Geometry: see drawing. Coordinates: mm, zero at the bounding-box minimum. A direction names the side the tool comes from. Give positions to 0.01 mm unless a question says otherwise; leave off trailing zeros. Loops run counter-clockwise (first coordinate to the right, second up) from the corner with the lowest first, then second, coordinate; pieces in that order, holes last. Notation, with made-up numbers: M 63,-12.75 L 100,-12.75 A22 cw 100,16.25 Z; hole C 77,-1 d3. An arc over 180 degrees is marked long. Answer in a Markdown table with one row per item.
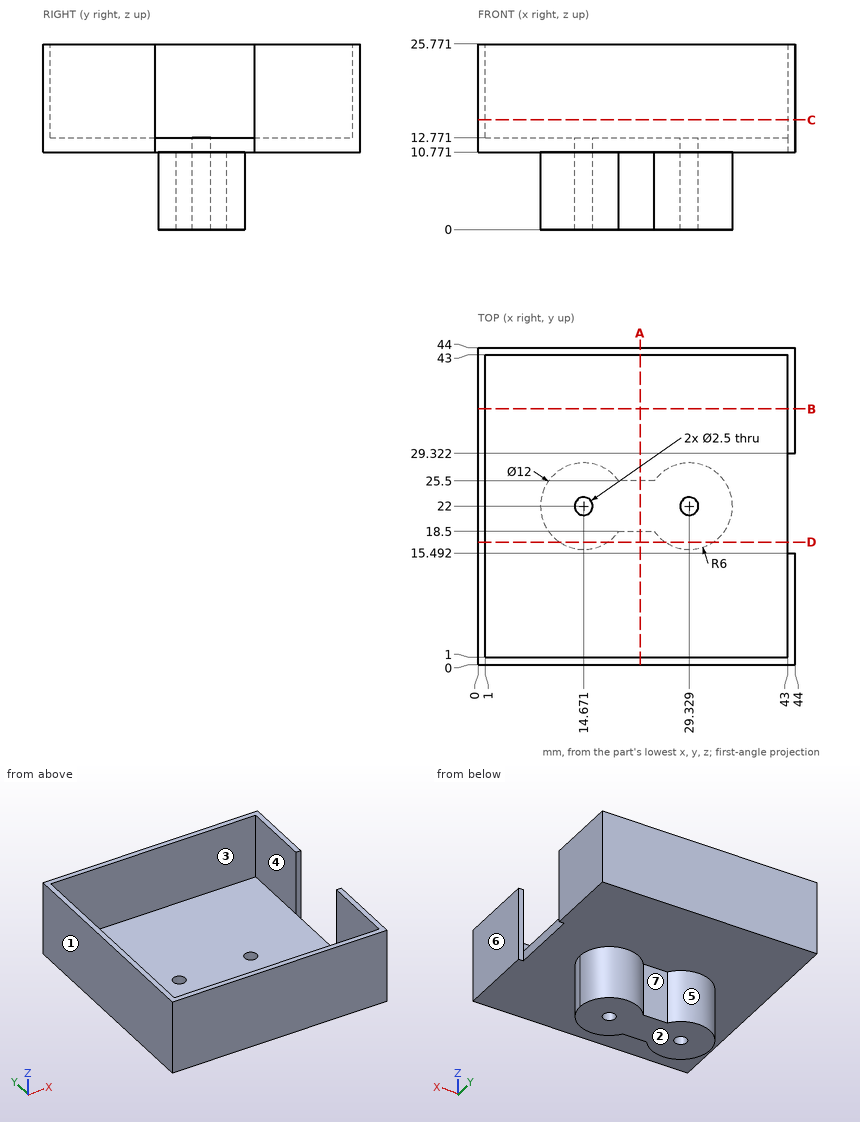
1) Section B-B, the plane y = 35.5. Return loops of the section in (x, z).
Reply:
| item | result |
|---|---|
| outline | M 0,10.77 L 44,10.77 L 44,25.77 L 43,25.77 L 43,12.77 L 1,12.77 L 1,25.77 L 0,25.77 Z |
2) Material intervals for L1, parallel to X at y = 22, z = 3.5; L2, parallel to X at y = 12, z = 14.75, sorted ascending.
Reply:
| item | result |
|---|---|
| L1 | x = 8.67 to 13.42, 15.92 to 28.08, 30.58 to 35.33 |
| L2 | x = 0 to 1, 43 to 44 |
3) Section A-A, the plane x = 22.5. Return loops of the section in (y, z).
Reply:
| item | result |
|---|---|
| outline | M 0,10.77 L 18.5,10.77 L 18.5,0 L 25.5,0 L 25.5,10.77 L 44,10.77 L 44,25.77 L 43,25.77 L 43,12.77 L 1,12.77 L 1,25.77 L 0,25.77 Z |
4) Section D-D, the plane y = 17. Return loops of the section in (x, z) (1 decimal), then the cut area to 3 significant figures.
Reply:
| item | result |
|---|---|
| outline | M 0,10.8 L 11.4,10.8 L 11.4,0 L 18,0 L 18,10.8 L 26,10.8 L 26,0 L 32.6,0 L 32.6,10.8 L 43,10.8 L 43,12.8 L 1,12.8 L 1,25.8 L 0,25.8 Z |
| area | 242 mm² |
5) Pull-direction query (X, two-part tool) for the marked faces 1, 2 and 3; classes: released by +X, released by -X, zero draft, split by the parting line, or undercut.
Reply:
| item | result |
|---|---|
| face 1 | released by -X |
| face 2 | zero draft |
| face 3 | undercut |
6) Set-up query: the marked faces 4, 5, 6 and 7. Return all of +Z, -Z, +X, -X, +Y, -Y with unobstructed straight access to the full face (end or side cutting, diameter ignored); none if empty.
Reply:
| item | result |
|---|---|
| face 4 | +Z |
| face 5 | -Z |
| face 6 | +Z, -Z, +X, +Y, -Y |
| face 7 | -Z, +Y |
7) Section C-C, the plane z = 15.25. Return loops of the section in (x, y), then the cut area to 3 significant figures.
Reply:
| item | result |
|---|---|
| outline | M 0,0 L 44,0 L 44,15.49 L 43,15.49 L 43,1 L 1,1 L 1,43 L 43,43 L 43,29.32 L 44,29.32 L 44,44 L 0,44 Z |
| area | 158 mm² |
8) Pin query (flat end, axial travel): pin 1 Ø10 at (x, z) = (6.5, 4.5) entering from +Y; pin 2 Ø10 at (y, z) = (27.5, 5.5) entering from -X; pin 3 Ø0.6 at (y, z) = (21, 11.5) entering from +X. Return the tip coordinate at first contact, or that it passes through.
Reply:
| item | result |
|---|---|
| pin 1 | stops at y = 27.09 |
| pin 2 | stops at x = 8.69 |
| pin 3 | stops at x = 43 |
